```python
from build123d import *

# Parameters (mm, degrees)
F0_W      = 63
F0_H      = 93
F0_W_2    = 60
F0_H_2    = 90
F1_DEPTH  = 23
F2_W      = 13
F2_H      = 16
F3_DEPTH  = 25
F5_D      = 4
F5_DEPTH  = 12
F5_TIP    = 1.2017212381
F7_D      = 5
F7_DEPTH  = 12
F7_TIP    = 1.5021515476
F9_D      = 8
F9_DEPTH  = 12
F9_TIP    = 2.4034424761
F10_W     = 63
F10_H     = 93
F11_DEPTH = 1.5
F12_R     = 1.5
F13_DEPTH = 4
F14_SIZE  = 1.5


# Not quite as in the source:
# - a feature names something its author has since deleted; it is built from what else it names


with BuildPart() as f1:
    # F0 (on Top) → F1 (new body)
    with BuildSketch(Plane.XY):
        with Locations((30, 45)):
            Rectangle(F0_W, F0_H)
        with Locations((30, 45)):
            Rectangle(F0_W_2, F0_H_2, mode=Mode.SUBTRACT)
    extrude(amount=F1_DEPTH)

    # F2 (on face) → F3 (cut)
    with BuildSketch(Plane.XZ.offset(1.5)):
        with Locations((33.5, 8)):
            Rectangle(F2_W, F2_H)
    extrude(amount=-F3_DEPTH, mode=Mode.SUBTRACT)

    # F5
    with Locations(Plane.YZ.offset(61.5)):
        with Locations((51, 8), (66, 8), (36, 8), (21, 8)):
            Hole(F5_D / 2, depth=F5_DEPTH)
            with Locations((0, 0, -(F5_DEPTH + F5_TIP / 2))):  # 118° drill point
                Cone(0, F5_D / 2, F5_TIP, mode=Mode.SUBTRACT)

    # F7 (one way)
    with BuildSketch(Plane.XZ.offset(-90)):
        with Locations((13.5, 10), (38.5, 10)):
            Circle(F7_D / 2)
    extrude(amount=-F7_DEPTH, mode=Mode.SUBTRACT)
    with Locations(Plane.XZ.offset(-90)):
        with Locations((13.5, 10), (38.5, 10)):
            with Locations((0, 0, -(F7_DEPTH + F7_TIP / 2))):  # 118° drill point
                Cone(0, F7_D / 2, F7_TIP, mode=Mode.SUBTRACT)

    # F9
    with Locations(Plane(origin=(0, 91.5, 0), x_dir=(-1, 0, 0), z_dir=(0, 1, 0))):
        with Locations((-52.5, 16.5)):
            Hole(F9_D / 2, depth=F9_DEPTH)
            with Locations((0, 0, -(F9_DEPTH + F9_TIP / 2))):  # 118° drill point
                Cone(0, F9_D / 2, F9_TIP, mode=Mode.SUBTRACT)

    # F10 (on face) → F11 (join)
    with BuildSketch(Plane.XY.offset(23)):
        with Locations((30, 45)):
            Rectangle(F10_W, F10_H)
    extrude(amount=F11_DEPTH)

    # F12 (on face) → F13 (join)
    with BuildSketch(Plane(origin=(0, 0, 0), x_dir=(1, 0, 0), z_dir=(0, 0, -1))):
        with BuildLine():
            ThreePointArc((-1.5, -71.5), (-11.5, -81.5), (-1.5, -91.5))
            Line((-1.5, -91.5), (-1.5, -71.5))
        make_face()
        with Locations((-7.5, -81.5)):
            Circle(F12_R, mode=Mode.SUBTRACT)
        with BuildLine():
            Line((61.5, 1.5), (61.5, -18.5))
            ThreePointArc((61.5, -18.5), (71.5, -8.5), (61.5, 1.5))
        make_face()
        with Locations((67.5, -8.5)):
            Circle(F12_R, mode=Mode.SUBTRACT)
    extrude(amount=-F13_DEPTH)

    # F14
    f14_edges = [f1.edges().sort_by_distance(p)[0] for p in [
        (-9, 81.5, 4),
        (66, 8.5, 4),
    ]]
    chamfer(f14_edges, length=F14_SIZE)


solid = f1.part
```
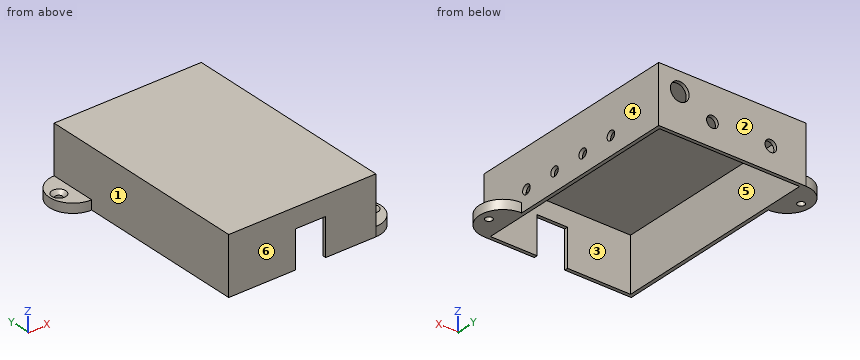
Can you work these out from the model? Positions are in its coordinate system, mm. Face numbers are marked on the shaded views. A direction names the side the tool comes from. Round coordinates to 2 decimals unless told otherwise and drop trailing zeros. Loops run counter-clockwise (first coordinate to the right, second up) from the corner with the lowest first, then second, coordinate; pieces in that order, holes last. Notation, with made-up numbers: M 75,-6 L 109,-6 A8 cw 109,3 Z; hole C -7.5,11 d8. An arc over 180 degrees is marked long. Write item = value, one per line. Start each with the question number.
(1) Suppose I cut it at A-A on x = -7.5. Write out the boundary of the cut face in (y, z).
(2) I'm going to push flat-ended pins straight in: P1, Ø2.5, axis at x = -7.5, y = 81.5, coming from the -Z side; P2, Ø3, axis at x = 67, y = 9, coming from the +Z side; P3, Ø1, axis at x = 28.5, y = 35, coming from the -Z side; P4, Ø0.8, axis at x = 30.5, y = -1, coming from the -Z side. Where does each tip first touch, or does it pass through?
(3) Suppose I cut it at B-B on y = 66. Write out the boundary of the cut face in (x, z), plus the area to 4 significant figures.
(4) Suppose I cut it at C-C on y = 28.5. Write out the boundary of the cut face in (x, z).
(5) Which directions (+Z, -Z, +X, -X, +Y, -Y) give clear straight access to the entire face, cutting with the end or side of a thin tool? Please do the marked faces 4, 5 and 6.
(6) I need wall thicknesses on line 1 along X through (y, z) = (54.5, 19); line 2 along Y through (x, z) = (41, 19.5); line 3 along Z through (x, y) = (43, 51). Which ranges of each line are inside material? Lowest first, please.
(7) If we mould it in two halves opening along Y, with no side actions, what happens to the marked faces 1, 2 and 3? For each: released by +Y, released by -Y, zero draft, split by the parting line, or undercut.
(8) Suppose I cut it at D-D on y = 8.5. Write out the boundary of the cut face in (x, z), plus the area to 3 significant figures.
Answer block:
q1.outline = M 73.5,0 L 80,0 L 80,2.5 L 78.5,4 L 73.5,4 Z; M 83,0 L 89.5,0 L 89.5,4 L 84.5,4 L 83,2.5 Z
q2.P1 = through
q2.P2 = 3.21
q2.P3 = 23
q2.P4 = 16
q3.outline = M -1.5,0 L 0,0 L 0,23 L 60,23 L 60,10 L 61.5,10 L 61.5,24.5 L -1.5,24.5 Z; M 60,0 L 61.5,0 L 61.5,6 L 60,6 Z
q3.area = 157.5 mm²
q4.outline = M -1.5,0 L 0,0 L 0,23 L 60,23 L 60,0 L 61.5,0 L 61.5,24.5 L -1.5,24.5 Z
q5.face_4 = +Z, +X, +Y
q5.face_5 = -Z
q5.face_6 = +Z, -Z, +X, -X, -Y
q6.line_1 = -1.5 to 0, 60 to 61.5
q6.line_2 = -1.5 to 0, 90 to 91.5
q6.line_3 = 23 to 24.5
q7.face_1 = zero draft
q7.face_2 = released by +Y
q7.face_3 = undercut
q8.outline = M -1.5,0 L 0,0 L 0,23 L 60,23 L 60,0 L 66,0 L 66,2.5 L 64.5,4 L 61.5,4 L 61.5,24.5 L -1.5,24.5 Z; M 69,0 L 71.5,0 L 71.5,4 L 70.5,4 L 69,2.5 Z
q8.area = 189 mm²
